Design review of the part built by this model. Coordinates are the model's own, in mm. Face numbers are marked on the shaded views. A direction names the side the tool comes from. Coordinates: 2 decimals unless noted, no trailing zeros. Loops run counter-clockwise (first coordinate to the right, second up) from the corner with the lowest first, then second, coordinate; pieces in that order, holes last. Notation, with made-up numbers: (-7, -4.75) - (27, -4.75) arc R21 cw to (27, 29.25) - close; hole circle Ø5 at (35, 78.25). An arc over 180 degrees is marked (long way). Answer in a Markdown table with one row per item. Add a question column.
(1) For the marked faces 1, 2, 3 and 4, list the 3-axis set-ups (+Z, -Z, +X, -X, +Y, -Y) from which the entire face can be reached by the end or side of a thin tool; tool diameter is ignored.
(2) We need section C-C, the plane y = -4.25. Write out the cut boundary in (x, z).
(3) We need section A-A, the plane z = 5.25. Write out the cut boundary in (x, y), plus the area to 3 significant figures.
(4) Clearance check with flat-ended pins moving along their axes: pin 1 (8.5 mm diameter, centred on x = -5, y = -9.5, fed in from -Z); pin 2 (14 mm diameter, centred on y = -8.5, z = -1, fed in from +X); pin 3 (2 mm diameter, centred on x = -1.5, y = 5.5, fed in from +Z); pin 4 (11 mm diameter, centred on x = -4.5, z = -4, fed in from +Y). State where each tip first meets the part, or that it passes through.
(5) We need section B-B, the plane x = 7. Write out the cut boundary in (y, z).
(6) We need section D-D, the plane x = 13. Write out the cut boundary in (y, z), plus the area to 3 significant figures.
(7) To check wall thickness, follow L1, parallel to X at y = -13.75, z = 5.5; L2, parallel to Z at x = 10, y = -7.25; L3, parallel to Y at x = -14, z = -8.5. State the ranges of each line that lie inside material, in increasing order. Write a range as [from, to].
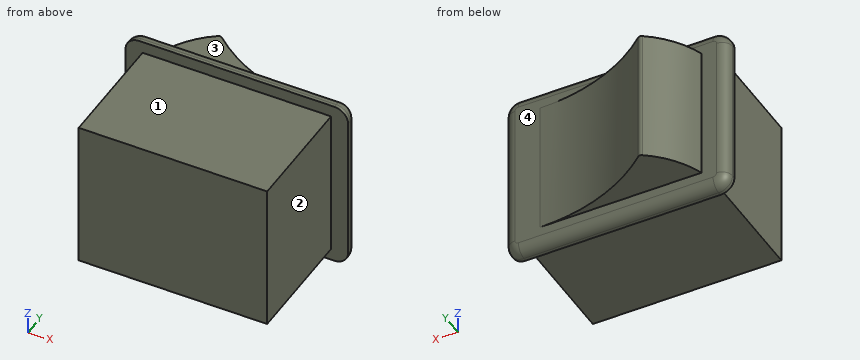
from build123d import *

# Parameters (mm, degrees)
BOSS_EXTRUDE1_DEPTH = 2
FILLET1_R           = 1.5
BOSS_EXTRUDE2_DEPTH = 9.75
SKETCH4_W           = 27.2
SKETCH4_H           = 17.2
BOSS_EXTRUDE3_DEPTH = 10.85


with BuildPart() as part:
    # Sketch1 → Boss-Extrude1 (new body)
    with BuildSketch(Plane(origin=(0, 0, 0), x_dir=(1, 0, 0), z_dir=(0, 1, 0))):
        with BuildLine():
            Line((-14.05, 12.6), (14.05, 12.6))
            ThreePointArc((14.05, 12.6), (15.464213562, 12.014213562), (16.05, 10.6))
            Line((16.05, 10.6), (16.05, -10.6))
            ThreePointArc((16.05, -10.6), (15.464213562, -12.014213562), (14.05, -12.6))
            Line((14.05, -12.6), (-14.05, -12.6))
            ThreePointArc((-14.05, -12.6), (-15.464213562, -12.014213562), (-16.05, -10.6))
            Line((-16.05, -10.6), (-16.05, 10.6))
            ThreePointArc((-16.05, 10.6), (-15.464213562, 12.014213562), (-14.05, 12.6))
        make_face()
    extrude(amount=BOSS_EXTRUDE1_DEPTH)

    # Fillet1
    fillet1_edges = [part.edges().sort_by_distance(p)[0] for p in [
        (-15.464213562, 2, -12.014213562),
        (-16.05, 2, 0),
        (-15.464213562, 2, 12.014213562),
        (0, 2, 12.6),
        (15.464213562, 2, 12.014213562),
        (16.05, 2, 0),
        (15.464213562, 2, -12.014213562),
        (0, 2, -12.6),
    ]]
    fillet(fillet1_edges, radius=FILLET1_R)

    # Sketch3 → Boss-Extrude2 (add, symmetric)
    with BuildSketch(Plane.XY):
        with BuildLine():
            Line((-12.369316877, 2), (10.942988923, 2))
            ThreePointArc((10.942988923, 2), (1.470491732, 3.716175191), (-6.79782289, 8.646533558))
            ThreePointArc((-6.79782289, 8.646533558), (-7.098799524, 8.768857552), (-7.4114107, 8.680402213))
            ThreePointArc((-7.4114107, 8.680402213), (-10.439168516, 5.747500287), (-12.369316877, 2))
        make_face()
    extrude(amount=BOSS_EXTRUDE2_DEPTH, both=True)

    # Sketch4 → Boss-Extrude3 (add, symmetric)
    with BuildSketch(Plane.XY):
        with Locations((0, -8.6)):
            Rectangle(SKETCH4_W, SKETCH4_H)
    extrude(amount=BOSS_EXTRUDE3_DEPTH, both=True)


solid = part.part
Responses:
| question | item | result |
|---|---|---|
| 1 | face 1 | +Z, +X, -X, -Y |
| 1 | face 2 | +Z, -Z, +X, -Y |
| 1 | face 3 | +Z, +X, -X, +Y |
| 1 | face 4 | +Y |
| 2 | outline | (-13.6, -10.85) - (13.6, -10.85) - (13.6, 10.85) - (-13.6, 10.85) - close |
| 3 | outline | (-16.05, 0) - (-13.6, 0) - (-13.6, -17.2) - (13.6, -17.2) - (13.6, 0) - (16.05, 0) - (16.05, 0.5) arc R1.5 ccw to (14.55, 2) - (10.94, 2) arc R27 cw to (-6.8, 8.65) arc R0.5 ccw to (-7.41, 8.68) arc R13 ccw to (-12.37, 2) - (-14.55, 2) arc R1.5 ccw to (-16.05, 0.5) - close |
| 3 | area | 593 mm2 |
| 4 | pin 1 | stops at z = -10.85 |
| 4 | pin 2 | stops at x = 13.6 |
| 4 | pin 3 | stops at z = 9.75 |
| 4 | pin 4 | stops at y = 8.77 |
| 5 | outline | (-17.2, -10.85) - (0, -10.85) - (0, -12.6) - (0.5, -12.6) arc R1.5 ccw to (2, -11.1) - (2, -9.75) - (2.29, -9.75) - (2.29, 9.75) - (2, 9.75) - (2, 11.1) arc R1.5 ccw to (0.5, 12.6) - (0, 12.6) - (0, 10.85) - (-17.2, 10.85) - close |
| 6 | outline | (-17.2, -10.85) - (0, -10.85) - (0, -12.6) - (0.5, -12.6) arc R1.5 ccw to (2, -11.1) - (2, 11.1) arc R1.5 ccw to (0.5, 12.6) - (0, 12.6) - (0, 10.85) - (-17.2, 10.85) - close |
| 6 | area | 423 mm2 |
| 7 | L1 | x = [-13.6, 13.6] |
| 7 | L2 | z = [-10.85, 10.85] |
| 7 | L3 | y = [0, 2] |
